Can you work these out from the model? Positions are in its coordinate system, mm. A direction names the side the tool comes from. Coordinates: 2 decimals unless noted, no trailing zeros. Loops run counter-clockwise (first coordinate to the right, second up) from the corner with the lowest first, then second, coordinate; pieces in that order, holes last. Notation, with made-up numbers: (8, 69.25) -> (48, 69.25) arc R29 ccw to (48, 106.25) -> close; hole circle Ø9 at (84.5, 41). An arc over 180 degrees is marked (long way). Put each result on its own line as item: value. Start each with the question number.
Item 1: For faces 1 (the flat face through (78.4, 2, 10)), 2 (the flat face through (114, 2, 15)), 3 (the flat face through (96, 2, 20)), which set-ups out of +Z, -Z, +X, -X, +Y, -Y let a thin tool reach every point of the face, with its end or its side?
Item 2: If we section it at A-A on z = 12.5: Please give me the cut outline in (x, y), plus the area to 3 significant figures.
Item 3: Will these pins go through, and if not, where does the flat tip stop? P1, Ø2.5, axis at x = 87, y = 3.5, coming from the +Z side; P2, Ø2.5, axis at y = 3.5, z = 17.5, coming from the +X side; P3, Ø3, axis at y = 1, z = 16, coming from the -X side; P4, Ø1.5, axis at y = 1.5, z = 17, coming from the -X side.
Item 4: If we section it at B-B on x = 39.5: Please give me the cut outline in (y, z).
Item 5: Please list where these lines run through material, in increasing order: L1, parallel to X at y = 3, z = 0; L2, parallel to Z at x = 83.5, y = 2.4; L3, parallel to X at y = 0.4, z = -0.5. Write a range as from..to.
Item 6: If we section it at C-C on z = -8: Please give me the cut outline in (x, y), plus the area to 3 significant figures.
Item 7: We'd pull the mould along X, two halves only. Please class faces 4 (the flat face through (125, 2, 8)), 5 (the flat face through (-23.5, 2, 17)), 6 (the flat face through (-103.5, 2, 17)), 7 (the flat face through (-64, 2, 20)): pulls with the +X half, pulls with the -X half, needs draft (parallel to the pull), parting line crosses it, or undercut.
```python
from build123d import *

# Parameters (mm, degrees)
EXTRUDE_1_DEPTH = 5


with BuildPart() as part:
    # 草圖1 → 填料-伸長1 (new body)
    with BuildSketch(Plane(origin=(0, 0, 0), x_dir=(1, 0, 0), z_dir=(0, 1, 0))):
        Polygon((-125, -15), (-103.5, -15), (-103.5, -20), (-88.5, -20), (-88.5, -15), (-81.6, -15), (-81.6, -5), (-85, -5), (-85, -2), (-81.6, -2), (-81.6, 2), (-78.4, 2), (-78.4, -2), (-75, -2), (-75, -5), (-78.4, -5), (-78.4, -15), (-71.5, -15), (-71.5, -20), (-56.5, -20), (-56.5, -15), (-23.5, -15), (-23.5, -20), (-8.5, -20), (-8.5, -15), (-1.6, -15), (-1.6, -5), (-5, -5), (-5, -2), (-1.6, -2), (-1.6, 1), (1.6, 1), (1.6, -2), (5, -2), (5, -5), (1.6, -5), (1.6, -15), (8.5, -15), (8.5, -20), (23.5, -20), (23.5, -15), (56.5, -15), (56.5, -20), (71.5, -20), (71.5, -15), (78.4, -15), (78.4, -5), (75, -5), (75, -2), (78.4, -2), (78.4, 2), (81.6, 2), (81.6, -2), (85, -2), (85, -5), (81.6, -5), (81.6, -15), (88.5, -15), (88.5, -20), (103.5, -20), (103.5, -15), (125, -15), (125, 0), (105, 15), (-105, 15), (-125, 0), align=None)
    extrude(amount=EXTRUDE_1_DEPTH)


solid = part.part
```
Solutions:
1. face 1: +Z, +Y, -Y
1. face 2: +Z, +X, +Y, -Y
1. face 3: +Z, +X, -X, +Y, -Y
2. outline: (-125, 0) -> (-81.6, 0) -> (-81.6, 5) -> (-125, 5) -> close; (-78.4, 0) -> (-1.6, 0) -> (-1.6, 5) -> (-78.4, 5) -> close; (1.6, 0) -> (78.4, 0) -> (78.4, 5) -> (1.6, 5) -> close; (81.6, 0) -> (125, 0) -> (125, 5) -> (81.6, 5) -> close
2. area: 1,200 mm^2
3. P1: z = 15
3. P2: x = 103.5
3. P3: x = -125
3. P4: x = -103.5
4. outline: (0, -15) -> (5, -15) -> (5, 15) -> (0, 15) -> close
5. L1: -125..-81.6, -78.4..-1.6, 1.6..78.4, 81.6..125
5. L2: -15..2, 5..15
5. L3: -124.33..-81.6, -78.4..-1.6, 1.6..78.4, 81.6..124.33
6. outline: (-114.33, 0) -> (114.33, 0) -> (114.33, 5) -> (-114.33, 5) -> close
6. area: 1,140 mm^2
7. face 4: pulls with the +X half
7. face 5: undercut
7. face 6: pulls with the -X half
7. face 7: needs draft
